The listing builds one solid part. Answer for the finished solid, in the listing's coordinates (mm). Face numbers are marked on the shaded views. A direction names the side the tool comes from. Give positions to 0.01 mm unless a question says otherwise; leave off trailing zeros. Write each loop counter-clockwise with the first axis right and the second up, starting at its lowest first coordinate (ties: lowest second). Pieces come first, ordered by that corner, then holes. Notation, with made-up numbers: (-28, 82.5) - (-21, 82.5) arc R29 ccw to (-21, 114.5) - close; hole circle Ø2 at (19, 34.25). An arc over 180 degrees is marked (long way). Return JSON: item names as keys, results as strings.
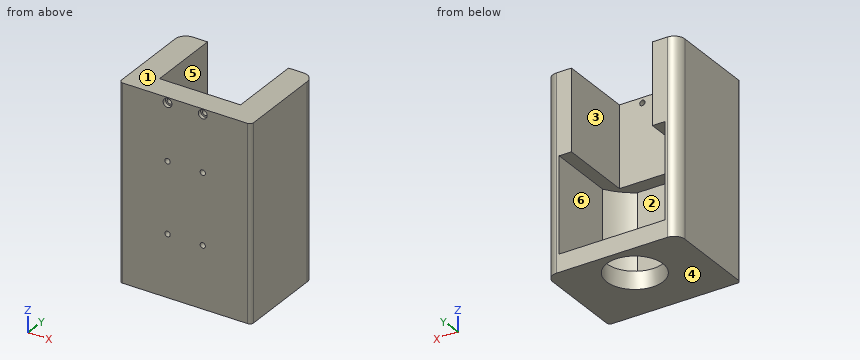
Autodesk Inventor part; units mm, degrees
ref_plane "YZ Plane" through (0, 0, 0) normal (1, 0, 0) x (0, 1, 0)
ref_plane "XZ Plane" through (0, 0, 0) normal (0, 1, 0) x (-1, 0, 0)
ref_plane "XY Plane" through (0, 0, 0) normal (0, 0, 1) x (1, 0, 0)
sketch "Sketch1" plane through (0, 0, 0) normal (0, 1, 0) x (-1, 0, 0)
  line L0 (0, 0) -> (75, 0)
  line L1 (75, 0) -> (75, -91)
  line L2 (75, -91) -> (0, -91)
  line L3 (0, -91) -> (0, 0)
  dimension "d0" = 75
  dimension "d1" = 91
extrude "Extrusion1" add sketch "Sketch1" along normal blind 5
sketch "Sketch2" plane through (0, 5, 0) normal (0, 1, 0) x (1, 0, 0)
  line L0 (-14.5, 42) -> (0, 42)
  line L1 (0, 0) -> (0, 91)
  line L2 (0, 42) -> (0, 0)
  line L3 (0, 0) -> (-14.5, 0)
  line L4 (0, 91) -> (-75, 91)
  line L5 (-60.5, 42) -> (-75, 42)
  line L6 (-75, 42) -> (-75, 0)
  line L7 (-75, 0) -> (-60.5, 0)
  line L8 (-60.5, 42) -> (-14.5, 42)
  line L9 (-14.5, 0) -> (-60.5, 0)
  line L10 (-75, 0) -> (0, 0)
extrude "Extrusion2" add sketch "Sketch2" along normal blind 8
sketch "Sketch3" plane through (0, 0, -91) normal (0, 0, -1) x (-1, 0, 0)
  line L0 (0, 5) -> (75, 5)
  line L1 (75, 0) -> (0, 0)
  line L2 (0, 5) -> (75, 5)
  line L3 (75, 5) -> (75, 0)
  line L4 (75, 0) -> (0, 0)
  line L5 (0, 0) -> (0, 5)
extrude "Extrusion3" add sketch "Sketch3" along normal blind 15
sketch "Sketch4" plane through (0, 13, 0) normal (0, 1, 0) x (1, 0, 0)
  line L0 (-14.5, 0) -> (-14.5, 42)
  line L1 (0, 42) -> (-75, 42)
  line L2 (-60.5, 0) -> (-60.5, 42)
  line L3 (-75, 0) -> (0, 0)
  line L4 (0, 0) -> (-14.5, 0)
  line L5 (-14.5, 0) -> (-14.5, 42)
  line L6 (-14.5, 42) -> (0, 42)
  line L7 (0, 42) -> (0, 0)
  line L8 (-60.5, 42) -> (-75, 42)
  line L9 (-75, 42) -> (-75, 0)
  line L10 (-75, 0) -> (-60.5, 0)
  line L11 (-60.5, 0) -> (-60.5, 42)
extrude "Extrusion4" add sketch "Sketch4" along normal blind 42 contours L0 L1 L7 L3 | L3 L9 L1 L2
sketch "Sketch5" plane through (0, 0, -106) normal (0, 0, -1) x (-1, 0, 0)
  line L0 (75, 5) -> (0, 5)
  line L1 (37.5, 5) -> (19.472, 5)
  line L2 (19.472, 5) -> (55.528, 5)
  line L3 (37.5, 5) -> (37.5, 35)
  line L4 (75, 0) -> (75, 55)
  line L5 (0, 5) -> (0, 55)
  line L6 (37.5, 35) -> (7.5, 35)
  line L7 (67.5, 35) -> (67.5, 16.972)
  line L8 (67.5, 35) -> (67.5, 53.028)
  arc A0 (55.528, 5) -> (67.5, 16.972) centre (37.5001, 34.9999) ccw
  line L9 (7.5, 35) -> (7.5, 53.028)
  line L10 (7.5, 35) -> (7.5, 16.9723)
  arc A1 (7.5, 16.9723) -> (19.472, 5) centre (37.5014, 35.001) ccw
  line L11 (67.5, 53.028) -> (75, 53.028)
  line L12 (75, 0) -> (0, 0)
  line L13 (75, 53.028) -> (75, 0)
  line L14 (75, 0) -> (0, 0)
  line L15 (0, 0) -> (0, 53.028)
  line L16 (7.5, 53.028) -> (0, 53.028)
  dimension "d18" = 18.028
  dimension "d19" = 36.056
  dimension "d20" = 30
  dimension "d21" = 30
  dimension "d22" = 30
  dimension "d23" = 18.028
  dimension "d24" = 18.028
  dimension "d25" = 35
extrude "Extrusion5" add sketch "Sketch5" against normal up to surface (64 mm away) contours L0 A0 L7 L8 L11 L4 | L0 L5 L16 L9 L10 A1
sketch "Sketch6" plane through (-75, 0, 0) normal (0, 0, 1) x (1, 0, 0)
  line L0 (0, 0) -> (0, 55)
  line L1 (75, 0) -> (0, 0)
  line L2 (0, 55) -> (0, 0)
  line L3 (0, 0) -> (75, 0)
  line L4 (75, 53.028) -> (75, 55)
  line L5 (75, 0) -> (75, 55)
  line L6 (75, 55) -> (60.5, 55)
  line L7 (75, 55) -> (60.5, 55)
  line L8 (60.5, 13) -> (60.5, 55)
  line L9 (60.5, 55) -> (60.5, 13)
  line L10 (60.5, 13) -> (14.5, 13)
  line L11 (60.5, 13) -> (14.5, 13)
  line L12 (14.5, 13) -> (14.5, 55)
  line L13 (14.5, 13) -> (14.5, 55)
  line L14 (14.5, 55) -> (0, 55)
extrude "Extrusion6" add sketch "Sketch6" along normal blind 4
sketch "Sketch8" plane through (0, 0, 0) normal (0, -1, 0) x (1, 0, 0)
  line L0 (-14.5, 4) -> (-60.5, 4)
  point P0 (0, 0)
  point P1 (-27.5, 1)
  point P2 (-47.5, 1)
hole "Hole2" at (-27.5, 0, 1) at (-47.5, 0, 1) direction (0, 1, 0) diameter 3 end through all counterbore diameter 5 counterbore depth 2
sketch "Sketch9" plane through (0, 55, 0) normal (0, 1, 0) x (1, 0, 0)
  point P0 (0, 0)
sketch "Sketch10" plane through (0, 5, 0) normal (0, 1, 0) x (1, 0, 0)
  line L0 (-67.5, 106) -> (-67.5, 42)
  line L1 (-7.5, 106) -> (-67.5, 106)
  line L2 (-67.5, 106) -> (-67.5, 96)
  line L3 (-67.5, 96) -> (-7.5, 96)
  line L4 (-7.5, 106) -> (-7.5, 42)
  line L5 (-7.5, 96) -> (-7.5, 106)
  point P0 (0, 0)
  dimension "d50" = 10
extrude "Extrusion7" add sketch "Sketch10" along normal up to surface (48.028 mm away)
sketch "Sketch11" plane through (0, 0, -106) normal (0, 0, -1) x (-1, 0, 0)
  line L0 (55.528, 5) -> (19.472, 5)
  circle A0 centre (37.5, 35) radius 16.5
  point P0 (0, 0)
  dimension "d56" = 33
extrude "Extrusion8" cut sketch "Sketch11" against normal through all
sketch "Sketch12" plane through (-75, 53.028, -106) normal (0, 1, 0) x (1, 0, 0)
  line L0 (75, -64) -> (67.5, -64)
  line L1 (75, 0) -> (75, -64)
  line L2 (75, -64) -> (75, 0)
  line L3 (75, 0) -> (0, 0)
  line L4 (75, 0) -> (0, 0)
  line L5 (7.5, -64) -> (0, -64)
  line L6 (0, 0) -> (0, -64)
  line L7 (7.5, -10) -> (7.5, -64)
  line L8 (0, -64) -> (7.5, -64)
  line L9 (7.5, -64) -> (7.5, -10)
  line L10 (67.5, -10) -> (7.5, -10)
  line L11 (7.5, -10) -> (67.5, -10)
  line L12 (67.5, -10) -> (67.5, -64)
  line L13 (67.5, -10) -> (67.5, -64)
  line L14 (67.5, -64) -> (75, -64)
  point P0 (75, -106)
extrude "Extrusion9" add sketch "Sketch12" along normal up to surface (1.972 mm away)
fillet "Fillet2" radius 2 2 edges at (0, 0, -51) (-75, 0, -51)
fillet "Fillet3" radius 6 2 edges at (0, 55, -51) (-75, 55, -51)
sketch "Sketch13" plane through (0, 0, 0) normal (0, -1, 0) x (1, 0, 0)
  line L0 (-2, 4) -> (-2, -106)
  line L1 (-73, -106) -> (-73, 4)
  circle A0 centre (-27.5, -31) radius 1.5
  circle A1 centre (-47.5, -31) radius 1.5
  circle A2 centre (-47.5, -71) radius 1.5
  circle A3 centre (-27.5, -71) radius 1.5
  point P0 (0, 0)
  dimension "d68" = 3
extrude "Extrusion10" cut sketch "Sketch13" against normal blind 10
sketch "Sketch14" plane through (0, 0, -106) normal (0, 0, -1) x (-1, 0, 0)
  circle A0 centre (37.5, 35) radius 16.5
  circle A1 centre (37.5, 35) radius 16
  point P0 (0, 0)
  dimension "d71" = 32
extrude "Extrusion11" add sketch "Sketch14" against normal up to surface (10 mm away)
properties part number "Motor_Mount"
Item 1: A cutting plane is placed at D-D on x = -37.5. Determine the outline of the cut face in (y, z).
Answer below:
{"outline": "(0, -106) - (19, -106) - (19, -96) - (5, -96) - (5, -42) - (13, -42) - (13, 4) - (0, 4) - close; (51, -106) - (55, -106) - (55, -96) - (51, -96) - close"}
Item 2: The mould has two halves that part along Z. Classify the marked faces 1, 2 and 3: +Z half, -Z half, draft (parallel to the pull), parting line (faces both ways), or undercut.
Answer below:
{"face 1": "+Z half", "face 2": "undercut", "face 3": "draft"}
Item 3: A cutting plane is placed at A-A on x = -27.5. Determine the outline of the cut face in (y, z).
Answer below:
{"outline": "(0, -106) - (22.51, -106) - (22.51, -96) - (5, -96) - (5, -72.5) - (0, -72.5) - close; (0, -69.5) - (5, -69.5) - (5, -42) - (13, -42) - (13, -0.5) - (2, -0.5) - (2, -1.5) - (0, -1.5) - (0, -29.5) - (10, -29.5) - (10, -32.5) - (0, -32.5) - close; (0, 3.5) - (2, 3.5) - (2, 2.5) - (13, 2.5) - (13, 4) - (0, 4) - close; (47.49, -106) - (55, -106) - (55, -96) - (47.49, -96) - close"}
Item 4: Flat-ended cylindrical pins translate along their axes: P1, Ø1.5, axis at x = -46.5, z = 1, coming from the -Y side; P2, Ø10, axis at x = -43.5, z = -81, coming from the -Y side; P3, Ø2.5, axis at x = -27.5, z = 1, coming from the -Y side; P4, Ø6, axis at x = -21.5, z = -12, coming from the +Y side. Find the tip coordinate at first contact, or state that the pin passes through.
Answer below:
{"P1": "stops at y = 2", "P2": "stops at y = 0", "P3": "passes through", "P4": "stops at y = 13"}
Item 5: For the marked faces 4, 5 and 6, determine the directions among +Z, -Z, +X, -X, +Y, -Y from which every point of the face is accessible in a straight line to the end or side of a thin tool.
Answer below:
{"face 4": "-Z, +X, -X, +Y, -Y", "face 5": "+Z, +Y", "face 6": "+Y"}
Item 6: A cutting plane is placed at B-B on z = 1. Determine the outline of the cut face in (x, y), then the cut area to 3 significant figures.
Answer below:
{"outline": "(-75, 2) arc R2 ccw to (-73, 0) - (-50, 0) - (-50, 2) - (-49, 2) - (-49, 13) - (-60.5, 13) - (-60.5, 55) - (-69, 55) arc R6 ccw to (-75, 49) - close; (-46, 2) - (-45, 2) - (-45, 0) - (-30, 0) - (-30, 2) - (-29, 2) - (-29, 13) - (-46, 13) - close; (-26, 2) - (-25, 2) - (-25, 0) - (-2, 0) arc R2 ccw to (0, 2) - (0, 49) arc R6 ccw to (-6, 55) - (-14.5, 55) - (-14.5, 13) - (-26, 13) - close", "area": "2,090 mm²"}
Item 7: A cutting plane is placed at C-C on y = 31. Determine the outline of the cut face in (x, z).
Answer below:
{"outline": "(-75, -106) - (-52.99, -106) - (-52.99, -96) - (-67.5, -96) - (-67.5, -42) - (-60.5, -42) - (-60.5, 4) - (-75, 4) - close; (-22.01, -106) - (0, -106) - (0, 4) - (-14.5, 4) - (-14.5, -42) - (-7.5, -42) - (-7.5, -96) - (-22.01, -96) - close"}
Item 8: Consider L1, parallel to Z at x = -47.5, y = 0.75; L2, parallel to Z at x = -47.5, y = 2.45; L3, parallel to X at y = 5.5, z = 1. Determine where each line is inside the solid, lowest interval first.
Answer below:
{"L1": "z = -106 to -72.5, -69.5 to -32.5, -29.5 to -1.5, 3.5 to 4", "L2": "z = -106 to -72.5, -69.5 to -32.5, -29.5 to -0.5, 2.5 to 4", "L3": "x = -75 to -49, -46 to -29, -26 to 0"}
